Could you check a few things on this model? Use its own coordinates, in mm. Coordinates: 2 decimals unless noted, no trailing zeros. Write each loop counter-clockwise with the first axis right and the second up, starting at its lowest first coordinate (ties: lowest second). Pieces come first, ordered by that corner, then holes.
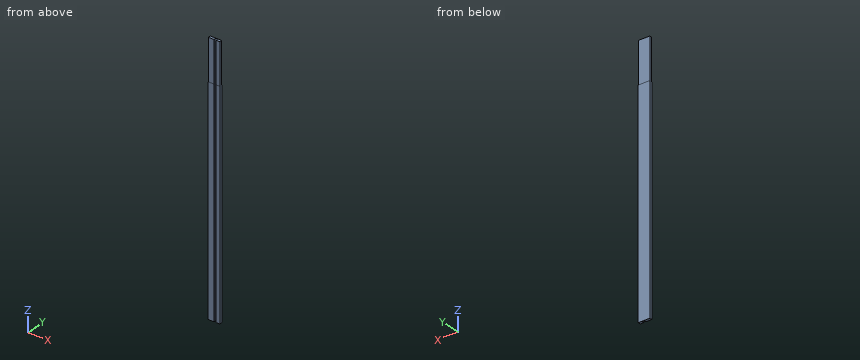
```python
from build123d import *

# Parameters (mm, degrees)
SKETCH1_W           = 25
SKETCH1_H           = 5.5
EXTRUDE1_DEPTH      = 259.4
SKETCH6_W           = 25
SKETCH6_H           = 20
BOSS_EXTRUDE2_DEPTH = 5.5
CUT_EXTRUDE2_DEPTH  = 559.8
SKETCH8_W           = 88.25
SKETCH8_H           = 0.06858
CUT_EXTRUDE3_DEPTH  = 26


with BuildPart() as part:
    # Sketch1 → Extrude1 (new body, symmetric)
    with BuildSketch(Plane.XY):
        Rectangle(SKETCH1_W, SKETCH1_H)
    extrude(amount=EXTRUDE1_DEPTH, both=True)

    # Sketch6 → Boss-Extrude2 (add)
    with BuildSketch(Plane(origin=(0, 2.75, 0), x_dir=(1, 0, 0), z_dir=(0, 1, 0))):
        with Locations((0, 269.4)):
            Rectangle(SKETCH6_W, SKETCH6_H)
        with Locations((0, -269.4)):
            Rectangle(SKETCH6_W, SKETCH6_H)
    extrude(amount=-BOSS_EXTRUDE2_DEPTH)

    # Sketch7 → Cut-Extrude2 (cut, through all)
    with BuildSketch(Plane.XY.offset(279.4)):
        with BuildLine():
            Line((-0.00025, -0.1278), (-0.00025, -2.75))
            Line((-0.00025, -2.75), (4.76225, -2.75))
            Line((4.76225, -2.75), (4.76225, -0.1278))
            ThreePointArc((4.76225, -0.1278), (2.381, 2.25345), (-0.00025, -0.1278))
        make_face()
    extrude(amount=-CUT_EXTRUDE2_DEPTH, mode=Mode.SUBTRACT)

    # Sketch8 → Cut-Extrude3 (cut, through all)
    with BuildSketch(Plane.ZY.offset(12.5)):
        with Locations((235.275, 2.71571)):
            Rectangle(SKETCH8_W, SKETCH8_H)
        with Locations((235.275, -2.71571)):
            Rectangle(SKETCH8_W, SKETCH8_H)
    extrude(amount=-CUT_EXTRUDE3_DEPTH, mode=Mode.SUBTRACT)


solid = part.part
```
1. I want a section at B-B on z = -29. Please give me the cut outline in (x, y).
Verdict:
outline: (-12.5, -2.75) - (0, -2.75) - (0, -0.13) arc R2.38 cw to (4.76, -0.13) - (4.76, -2.75) - (12.5, -2.75) - (12.5, 2.75) - (-12.5, 2.75) - close
2. Please list where these lines run through material, in increasing order: line 1 along X through (y, z) = (-2.4, 126.5); line 2 along Y through (x, z) = (6, 217.5); line 3 along X through (y, z) = (0.7, -75.5).
Verdict:
line 1: x = -12.5 to 0, 4.76 to 12.5
line 2: y = -2.68 to 2.68
line 3: x = -12.5 to 0.15, 4.61 to 12.5
3. For pin 1 (3.5 mm diameter, centred on x = -8, z = 245, fed in from -Y), with a flat end and sliding along its axis, tell me the tip position at first contact or that it passes through.
Verdict:
pin 1: stops at y = -2.68
4. I want a section at A-A on y = -1.8. Please give me the cut outline in (x, z), plus the area to 3 significant figures.
Verdict:
outline: (-12.5, -279.4) - (0, -279.4) - (0, 279.4) - (-12.5, 279.4) - close; (4.76, -279.4) - (12.5, -279.4) - (12.5, 279.4) - (4.76, 279.4) - close
area: 11,300 mm2
